```python
from build123d import *

# Parameters (mm, degrees)
F1_DEPTH      = 150
F1_DEPTH_BACK = 150


with BuildPart() as f1:
    # F0 (on Right) → F1 (new body, two sides)
    with BuildSketch(Plane.YZ) as f1_sk:
        Polygon((-11.5, -1.5), (11.5, -1.5), (11.5, 1.5), (1.5, 1.5), (1.5, 26.5), (14.5, 26.5), (14.5, 29.5), (14.5, 34.5), (17.5, 34.5), (17.5, 37.5), (11.401065, 37.5), (7, 37.5), (7, 34.5), (11.401065, 34.5), (11.401065, 29.5), (-11.462442, 29.5), (-11.462442, 34.5), (-7, 34.5), (-7, 37.5), (-11.401065, 37.5), (-11.462442, 37.5), (-17.5, 37.5), (-17.5, 34.5), (-14.5, 34.5), (-14.5, 29.5), (-14.5, 26.5), (-1.5, 26.5), (-1.5, 1.5), (-11.5, 1.5), align=None)
    extrude(amount=F1_DEPTH)
    extrude(f1_sk.sketch, amount=-F1_DEPTH_BACK)


solid = f1.part
```
Model file for the job. Use its own axes, mm. A direction names the side the tool comes from. Round coordinates to 2 decimals unless told otherwise and drop trailing zeros. Order: outer loops, then holes, each group sorted by start corner. A loop starts at its lowest first (then second) coordinate and runs counter-clockwise, first axis right, second up. Notation, with made-up numbers: M -31.5,27.5 L 16.5,27.5 A14 cw 16.5,44.5 Z; hole C 66.5,-34 d10. An arc over 180 degrees is marked long. Use CSV: the item, a comma, the result in double quotes.
Item 1: Pin check, flat tips, straight feed: pin 1 (0.9 mm diameter, centred on x = 56.5, y = -16, fed in from -Z); pin 2 (12.5 mm diameter, centred on x = 70, z = 14, fed in from +Y); pin 3 (1.5 mm diameter, centred on x = -12.5, y = -2.5, fed in from +Z). Stop position of each tip, or through.
Worked answers:
pin 1,"z = 34.5"
pin 2,"y = 1.5"
pin 3,"z = 29.5"
Item 2: Saw through at A-A (z = 32). List the corners of the cut face in (x, y), plus the area to 3 significant figures.
Worked answers:
outline,"M -150,-14.5 L 150,-14.5 L 150,-11.46 L -150,-11.46 Z; M -150,11.4 L 150,11.4 L 150,14.5 L -150,14.5 Z"
area,"1,840 mm²"
Item 3: Saw through at C-C (z = 20). List the corners of the cut face in (x, y).
Worked answers:
outline,"M -150,-1.5 L 150,-1.5 L 150,1.5 L -150,1.5 Z"
Item 4: Which spindle directions (+Z, -Z, +X, -X, +Y, -Y) get a long thin tool onto all of the face, cutting with end or side? Do faces 4 (the face through (2, -1.5, 14)), 5 (the face through (2, 1.5, 14)), 6 (the face through (2, -11.462, 32)). Say none if no direction does.
Worked answers:
face 4,"+X, -X, -Y"
face 5,"+X, -X, +Y"
face 6,"+X, -X"
Item 5: Probe probe 1 along Y at (x, z) = (127.5, 30); probe 2 along Y at (x, z) = (61.5, 36); probe 3 along Z at (x, y) = (-48, -5.5). List the from-to ranges inside material, lowest first.
Worked answers:
probe 1,"-14.5 to -11.46, 11.4 to 14.5"
probe 2,"-17.5 to -7, 7 to 17.5"
probe 3,"-1.5 to 1.5, 26.5 to 29.5"
Item 6: Pull direction Z, two halves, no side cores. Call faces 1 (the face through (2, -14.5, 31)), 2 (the face through (2, 0, -1.5)), 3 (the face through (2, 7, 1.5)): released by +Z, released by -Z, zero draft, split by the parting line, or undercut.
Worked answers:
face 1,"zero draft"
face 2,"released by -Z"
face 3,"undercut"
Item 7: Saw through at B-B (x = 130). List the corners of the cut face in (y, z), plus the area to 3 significant figures.
Worked answers:
outline,"M -17.5,34.5 L -14.5,34.5 L -14.5,26.5 L -1.5,26.5 L -1.5,1.5 L -11.5,1.5 L -11.5,-1.5 L 11.5,-1.5 L 11.5,1.5 L 1.5,1.5 L 1.5,26.5 L 14.5,26.5 L 14.5,34.5 L 17.5,34.5 L 17.5,37.5 L 7,37.5 L 7,34.5 L 11.4,34.5 L 11.4,29.5 L -11.46,29.5 L -11.46,34.5 L -7,34.5 L -7,37.5 L -17.5,37.5 Z"
area,"325 mm²"
